Geometry check sheet. Reference: drawing and pictorial views, mm from the part's lowest x, y, z. A direction names the side the tool comes from. Coordinates: 2 decimals unless noted, no trailing zeros. Write each loop counter-clockwise with the first axis right and the second up, starting at its lowest first coordinate (ties: lowest second). Pieces come first, ordered by that corner, then holes. Notation, with made-up numbers: (6.25, 85.5) -> (27.25, 85.5) arc R16 ccw to (27.25, 94.5) -> close; hole circle Ø9 at (-10.5, 49.5). An arc over 180 degrees is marked (long way). Put each result on its own line as item: value.
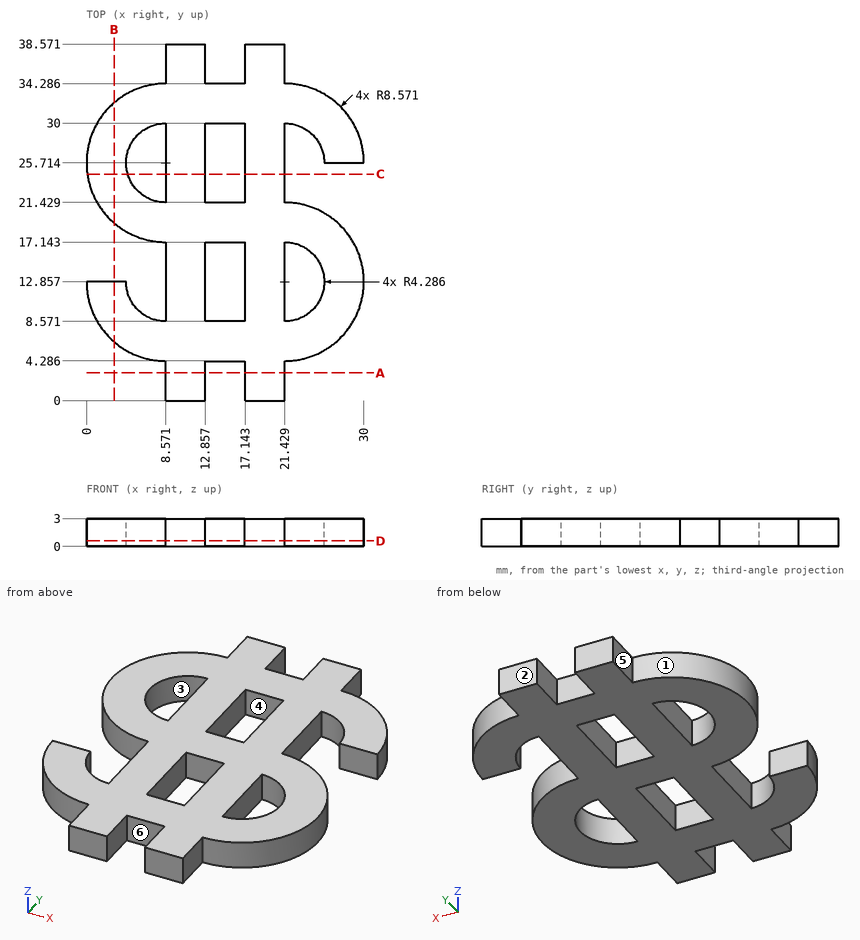
Q1. Cross-section at A-A (y = 3). Record the cut outline in (x, z), plus the area to 3 significant figures.
Recorded:
outline: (8.57, 0) -> (12.86, 0) -> (12.86, 3) -> (8.57, 3) -> close; (17.14, 0) -> (21.43, 0) -> (21.43, 3) -> (17.14, 3) -> close
area: 25.7 mm2
Q2. Depth check by flat-ended pin: P1, Ø1.5, axis at x = 9, z = 0.5, coming from the -Y side; P2, Ø0.9, axis at y = 27.5, z = 1, coming from the +X side (1 decimal); P3, Ø0.9, axis at x = 16, z = 2, coming from the +Y side; P4, Ø1.5, axis at y = 27.5, z = 2, coming from the -X side. Enter the tip coordinate at first touch or a pass-through.
Recorded:
P1: stops at y = 0
P2: stops at x = 29.9
P3: stops at y = 34.29
P4: stops at x = 0.06
Q3. Tool access check on the marked faces 4, 5 and 6. Record the directions out of +Z, -Z, +X, -X, +Y, -Y that give a thin tool (end or side, any length) a straight path to the whole face; none if there is none.
Recorded:
face 4: +Z, -Z
face 5: +Z, -Z, -X, +Y
face 6: +Z, -Z, -Y
Q4. Mould release check, pull along X, two halves, no side actions. Record for the marked faces 1, 2 and 3: released by +X, released by -X, zero draft, split by the parting line, or undercut.
Recorded:
face 1: released by -X
face 2: zero draft
face 3: undercut
Q5. Cross-section at B-B (x = 3). Record the cut outline in (y, z).
Recorded:
outline: (6.34, 0) -> (12.86, 0) -> (12.86, 3) -> (6.34, 3) -> close; (19.2, 0) -> (32.23, 0) -> (32.23, 3) -> (19.2, 3) -> close
Q6. Material ranges on line 1 along Y through (x, z) = (16.75, 2.3) (1 decimal); line 2 along X through (y, z) = (3, 2.6); line 3 along X through (y, z) = (16.5, 0.55) (1 decimal), recorded low to high.
Recorded:
line 1: y = 4.3 to 8.6, 17.1 to 21.4, 30 to 34.3
line 2: x = 8.57 to 12.86, 17.14 to 21.43
line 3: x = 8.6 to 12.9, 17.1 to 21.4, 23.7 to 29.2
Q7. Cross-section at C-C (y = 24.5). Record the cut outline in (x, z).
Recorded:
outline: (0.09, 0) -> (4.46, 0) -> (4.46, 3) -> (0.09, 3) -> close; (8.57, 0) -> (12.86, 0) -> (12.86, 3) -> (8.57, 3) -> close; (17.14, 0) -> (21.43, 0) -> (21.43, 3) -> (17.14, 3) -> close
Q8. Cross-section at D-D (z = 0.6). State how many separate pieces and enclosed holes the cut face has.
Recorded:
separate pieces: 1
enclosed holes: 4
